Part model, mm, in its own coordinate system. Face numbers are marked on the shaded views. A direction names the side the tool comes from. Give positions to 0.01 mm unless a question says otherwise; leave off trailing zeros. Write each loop counter-clockwise with the first axis right and the second up, starting at its lowest first coordinate (ties: lowest second). Pieces come first, ordered by that corner, then holes.
```python
from build123d import *

# Parameters (mm, degrees)
SKETCH_3_OUTSIDE_W   = 20.754
SKETCH_3_OUTSIDE_H   = 20.754
SKETCH_3_OUTSIDE_W_2 = 10
SKETCH_3_OUTSIDE_H_2 = 14.97891863
CUT_EXTRUDE_1_DEPTH  = 10


with BuildPart() as part:
    # 草图2 → 旋转1 (revolve)
    with BuildSketch(Plane(origin=(0, 0, 0), x_dir=(0, 0, -1), z_dir=(1, 0, 0))):
        Polygon((0, 0), (0, 6), (3, 6), (3, 4), (21.2, 4), (21.2, 3), (29.2, 3), (29.2, 0), align=None)
    revolve(axis=Axis((0, 0, 0), (0, 0, -1)))

    # 草图3 outside → 切除-拉伸1 (cut)
    with BuildSketch(Plane.XY):
        Rectangle(SKETCH_3_OUTSIDE_W, SKETCH_3_OUTSIDE_H)
        Rectangle(SKETCH_3_OUTSIDE_W_2, SKETCH_3_OUTSIDE_H_2, mode=Mode.SUBTRACT)
    extrude(amount=-CUT_EXTRUDE_1_DEPTH, mode=Mode.SUBTRACT)


solid = part.part
```
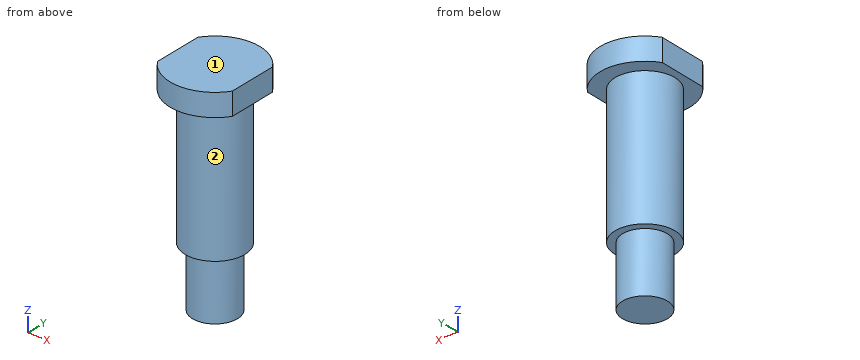
1) Saw through at C-C, the plane z = -24.75. Write the cut outline in (x, y), then the cut area to 3 significant figures.
Answers follow:
outline: circle Ø6 at (0, 0)
area: 28.3 mm2
2) Saw through at A-A, the plane y = 0. Write the cut outline in (x, z).
Answers follow:
outline: (-5, -3) - (-4, -3) - (-4, -21.2) - (-3, -21.2) - (-3, -29.2) - (3, -29.2) - (3, -21.2) - (4, -21.2) - (4, -3) - (5, -3) - (5, 0) - (-5, 0) - close
3) 3-axis set-ups, long thin cutter, end or side, ignore diameter. For the marked faces 1 and 2: which of +Z, -Z, +X, -X, +Y, -Y reach the whole face in a straight line?
Answers follow:
face 1: +Z, +X, -X, +Y, -Y
face 2: -Z
4) Saw through at D-D, the plane x = -3.5. Write the cut outline in (y, z).
Answers follow:
outline: (-4.87, -3) - (-1.94, -3) - (-1.94, -21.2) - (1.94, -21.2) - (1.94, -3) - (4.87, -3) - (4.87, 0) - (-4.87, 0) - close
5) Pin check, flat tips, straight feed: pin 1 Ø4 at (y, z) = (3.5, -5.5) entering from +X; pin 2 Ø5 at (x, z) = (1, -11.5) entering from -Y; pin 3 Ø2 at (y, z) = (-3, -15.5) entering from +X. Stop position of each tip, or through.
Answers follow:
pin 1: stops at x = 3.71
pin 2: stops at y = -4
pin 3: stops at x = 3.46
6) Saw through at B-B, the plane x = 0. Write the cut outline in (y, z), then the cut area to 3 significant figures.
Answers follow:
outline: (-6, -3) - (-4, -3) - (-4, -21.2) - (-3, -21.2) - (-3, -29.2) - (3, -29.2) - (3, -21.2) - (4, -21.2) - (4, -3) - (6, -3) - (6, 0) - (-6, 0) - close
area: 230 mm2
7) Wall check: L1, parallel to Z at x = -2, y = -4.5; L2, parallel to Z at x = 3, y = 1.5; L3, parallel to Y at x = -0.5, z = -10. Give the ranges that are in metal, low to high.
Answers follow:
L1: z = -3 to 0
L2: z = -21.2 to 0
L3: y = -3.97 to 3.97
